```python
from build123d import *

# Parameters (mm, degrees)
SKETCH_W     = 11.5
SKETCH_H     = 11.5
PAD_DEPTH    = 9.6
FILLET_R     = 1.4
SKETCH001_R  = 0.7
PAD001_DEPTH = 3.5


with BuildPart() as fillet_body:
    # Sketch → Pad (new body)
    with BuildSketch(Plane.XY.offset(0.1)):
        with Locations((3, 3)):
            Rectangle(SKETCH_W, SKETCH_H)
    extrude(amount=PAD_DEPTH)

    # Fillet
    fillet_edges = [fillet_body.edges().sort_by_distance(p)[0] for p in [
        (8.75, -2.75, 4.9),
        (8.75, 8.75, 4.9),
        (-2.75, -2.75, 4.9),
        (-2.75, 8.75, 4.9),
    ]]
    fillet(fillet_edges, radius=FILLET_R)


with BuildPart() as obj1:
    # Sketch001 → Pad001 (new body)
    with BuildSketch(Plane.XY.offset(0.5)):
        Circle(SKETCH001_R)
        with Locations((6, 6)):
            Circle(SKETCH001_R)
    extrude(amount=-PAD001_DEPTH)

    # obj1: union Fillet body
    add(fillet_body.part)


solid = obj1.part
```
Read the model definition and answer for the solid it produces. Units are mm, in the model's axes. A direction names the side the tool comes from. Coordinates: 2 decimals unless noted, no trailing zeros. Write each loop counter-clockwise with the first axis right and the second up, starting at its lowest first coordinate (ties: lowest second). Pieces come first, ordered by that corner, then holes. Notation, with made-up numbers: (14, 0) -> (68, 0) arc R21 cw to (68, 39) -> close; hole circle Ø8 at (67.5, 49.25). An arc over 180 degrees is marked (long way). Return JSON: item names as keys, results as strings.
1. A cutting plane is placed at D-D (y = 7). Determine the outline of the cut face in (x, z), and give its area (3 significant figures).
Found:
{"outline": "(-2.75, 0.1) -> (8.75, 0.1) -> (8.75, 9.7) -> (-2.75, 9.7) -> close", "area": "110 mm2"}
2. A cutting plane is placed at A-A (x = 0). Determine the outline of the cut face in (y, z), and give its area (3 significant figures).
Found:
{"outline": "(-2.75, 0.1) -> (-0.7, 0.1) -> (-0.7, -3) -> (0.7, -3) -> (0.7, 0.1) -> (8.75, 0.1) -> (8.75, 9.7) -> (-2.75, 9.7) -> close", "area": "115 mm2"}
3. A tool of negligible diameter and unlimited length cuts with its end or side. For faces 1 (the face through (5.48, 6.47, -1.43)), 2 (the face through (8.33, -2.35, 4.97)), from which of +Z, -Z, +X, -X, +Y, -Y can it reach the whole face along a straight path? Write none if from no direction.
Found:
{"face 1": "-Z", "face 2": "+Z, -Z, +X, -Y"}
4. A cutting plane is placed at B-B (z = -0.5). Determine the outline of the cut face in (x, y), and give its area (3 significant figures).
Found:
{"outline": "circle Ø1.4 at (0, 0); circle Ø1.4 at (6, 6)", "area": "3.08 mm2"}
5. Find the intervals of material crossed by line 1 along Z through (x, y) = (2, 0.25); line 2 along X through (y, z) = (-2, 0.25); line 3 along Y through (x, z) = (-1.75, 4.75), in increasing order. Write a range as from..to.
Found:
{"line 1": "0.1..9.7", "line 2": "-2.59..8.59", "line 3": "-2.69..8.69"}
6. This flat-tipped pin is pushed along its axis until it touches: P1, Ø1.5, axis at x = 5.5, y = 7.5, coming from the -Z side. Where does it stop, or does it pass through?
Found:
{"P1": "z = 0.1"}
